Verification items for the finished model (mm, model axes). A direction names the side the tool comes from. Give positions to 0.01 mm unless a question says otherwise; leave off trailing zeros. Order: outer loops, then holes, each group sorted by start corner. A loop starts at its lowest first (then second) coordinate and runs counter-clockwise, first axis right, second up. Notation, with made-up numbers: (77.5, -38.5) -> (135.5, -38.5) arc R26 cw to (135.5, -6.5) -> close; hole circle Ø9 at (53, 47.25). An arc over 180 degrees is marked (long way). Return JSON: item names as keys, results as strings. Group by question number.
(1) Tool access check on faces 5 (the face through (20, 0, 1)), 6 (the face through (12, 0, 1)). Record the directions out of +Z, -Z, +X, -X, +Y, -Y that give a thin tool (end or side, any length) a straight path to the whole face; none if there is none.
(2) Thickness scan on line 1 along Y through (x, z) = (-2.5, 1.6); line 2 along Y through (x, z) = (16, 1.5); line 3 along Y through (x, z) = (-13.75, 1.7). Record the ranges inside material, lowest first.
(3) Cross-section at B-B on x = 13.75. Enter the section's corners in (y, z).
(4) Cross-section at A-A on z = 1.9. Enter the section's corners in (x, y), then the cut area to 3 significant figures.
(5) Release check for a two-part mould opening along X. For faces 1 (the face through (0, 12.5, 1)), 2 (the face through (0, 6.75, 1)), 3 (the face through (-12, 0, 1)), 4 (the face through (-19.14, -11.6, 1.52)) record: pulls with the +X half, pulls with the -X half, needs draft (parallel to the pull), parting line crosses it, or undercut.
(6) Cross-section at C-C on y = 8.5. Enter the section's corners in (x, z), then the cut area to 3 significant figures.
(7) Depth check by flat-ended pin: pin 1 Ø1.2 at (x, y) = (-16, -8.5) entering from +Z. Enter the tip coordinate at first touch or a pass-through.
(8) Cross-section at D-D on y = -5.25. Enter the section's corners in (x, z), then the cut area to 3 significant figures.
from build123d import *

# Parameters (mm, degrees)
F0_R     = 1
F0_R_2   = 0.5
F0_W     = 24
F0_H     = 13.5
F1_DEPTH = 3
F2_R     = 3


with BuildPart() as f1:
    # F0 (on Top) → F1 (new body)
    with BuildSketch(Plane.XY):
        Polygon((20, -8.5), (20, 12.5), (16, 12.5), (-20, 12.5), (-20, -8.5), (-20, -12.5), (-16, -12.5), (16, -12.5), (20, -12.5), align=None)
        with Locations((-16, -8.5)):
            Circle(F0_R, mode=Mode.SUBTRACT)
        with Locations((16, -8.5)):
            Circle(F0_R, mode=Mode.SUBTRACT)
        with Locations((-13.75, 0)):
            Circle(F0_R_2, mode=Mode.SUBTRACT)
        with Locations((-16, 8.5)):
            Circle(F0_R, mode=Mode.SUBTRACT)
        Rectangle(F0_W, F0_H, mode=Mode.SUBTRACT)
        with Locations((13.75, 0)):
            Circle(F0_R_2, mode=Mode.SUBTRACT)
        with Locations((16, 8.5)):
            Circle(F0_R, mode=Mode.SUBTRACT)
    extrude(amount=F1_DEPTH)

    # F2
    f2_edges = [f1.edges().sort_by_distance(p)[0] for p in [
        (20, -12.5, 1.5),
        (-20, -12.5, 1.5),
        (20, 12.5, 1.5),
        (-20, 12.5, 1.5),
    ]]
    fillet(f2_edges, radius=F2_R)


solid = f1.part
Verdict:
{
 "1": {"face 5": "+Z, -Z, +X, +Y, -Y", "face 6": "+Z, -Z"},
 "2": {"line 1": "-12.5 to -6.75, 6.75 to 12.5", "line 2": "-12.5 to -9.5, -7.5 to 7.5, 9.5 to 12.5", "line 3": "-12.5 to -0.5, 0.5 to 12.5"},
 "3": {"outline": "(-12.5, 0) -> (-0.5, 0) -> (-0.5, 3) -> (-12.5, 3) -> close; (0.5, 0) -> (12.5, 0) -> (12.5, 3) -> (0.5, 3) -> close"},
 "4": {"outline": "(-20, -9.5) arc R3 ccw to (-17, -12.5) -> (17, -12.5) arc R3 ccw to (20, -9.5) -> (20, 9.5) arc R3 ccw to (17, 12.5) -> (-17, 12.5) arc R3 ccw to (-20, 9.5) -> close; hole circle Ø2 at (-16, -8.5); hole circle Ø2 at (-16, 8.5); hole circle Ø1 at (-13.75, 0); hole (-12, -6.75) -> (12, -6.75) -> (12, 6.75) -> (-12, 6.75) -> close; hole circle Ø1 at (13.75, 0); hole circle Ø2 at (16, -8.5); hole circle Ø2 at (16, 8.5)", "area": "654 mm²"},
 "5": {"face 1": "needs draft", "face 2": "undercut", "face 3": "undercut", "face 4": "pulls with the -X half"},
 "6": {"outline": "(-20, 0) -> (-17, 0) -> (-17, 3) -> (-20, 3) -> close; (-15, 0) -> (15, 0) -> (15, 3) -> (-15, 3) -> close; (17, 0) -> (20, 0) -> (20, 3) -> (17, 3) -> close", "area": "108 mm²"},
 "7": {"pin 1": "through"},
 "8": {"outline": "(-20, 0) -> (-12, 0) -> (-12, 3) -> (-20, 3) -> close; (12, 0) -> (20, 0) -> (20, 3) -> (12, 3) -> close", "area": "48.0 mm²"}
}
